Autodesk Inventor part; units mm, degrees
ref_plane "YZ Plane" through (0, 0, 0) normal (1, 0, 0) x (0, 1, 0)
ref_plane "XZ Plane" through (0, 0, 0) normal (0, 1, 0) x (-1, 0, 0)
ref_plane "XY Plane" through (0, 0, 0) normal (0, 0, 1) x (1, 0, 0)
sketch "Szkic1" plane through (0, 0, 0) normal (0, 0, 1) x (1, 0, 0)
  circle A0 centre (0, 0) radius 15
  circle A1 centre (0, 0) radius 5
  dimension "d0" = 30
  dimension "d1" = 10
extrude "Wyciągnięcie proste1" add sketch "Szkic1" along normal blind 14
sketch "Szkic2" plane through (0, 0, 14) normal (0, 0, 1) x (1, 0, 0)
  circle A0 centre (0, 0) radius 6.5
  circle A1 centre (0, 0) radius 13.5
  dimension "d4" = 13
  dimension "d5" = 27
extrude "Wyciągnięcie proste2" cut sketch "Szkic2" against normal blind 1
sketch "Szkic3" plane through (0, 0, 0) normal (0, 0, -1) x (-1, 0, 0)
  circle A0 centre (0, 0) radius 6.5
  circle A1 centre (0, 0) radius 13.5
  dimension "d8" = 13
  dimension "d9" = 27
extrude "Wyciągnięcie proste3" cut sketch "Szkic3" against normal blind 1
properties part number "Łożysko kulowe jednorzędowe 3200 2RS"
CAD build for the part. Positions are in the model's coordinates, mm. A direction names the side the tool comes from. Round coordinates to 2 decimals unless told otherwise and drop trailing zeros. Order: outer loops, then holes, each group sorted by start corner. A loop starts at its lowest first (then second) coordinate and runs counter-clockwise, first axis right, second up. Notation, with made-up numbers: (79.5, 44) -> (120.5, 44) arc R35 ccw to (120.5, 78) -> close; hole circle Ø8 at (68.5, 19.25). An arc over 180 degrees is marked (long way). Write item = value, one per line.
(1) Drill centre lines: L1, parallel to Y at x = 0, z = 13.65; L2, parallel to Y at x = 0, z = 7.25; L3, parallel to Z at x = -6.75, y = 6. Where is each one in solid material? Low to high.
Answers follow:
L1 = -15 to -13.5, -6.5 to -5, 5 to 6.5, 13.5 to 15
L2 = -15 to -5, 5 to 15
L3 = 1 to 13
(2) Cut at C-C (z = 5.75). Write the cut outline in (x, y), plus the area to 3 significant figures.
Answers follow:
outline = circle Ø30 at (0, 0); hole circle Ø10 at (0, 0)
area = 628 mm²
(3) Cut at D-D (x = -9.75). Write the cut outline in (y, z), plus the area to 3 significant figures.
Answers follow:
outline = (-11.4, 0) -> (-9.34, 0) -> (-9.34, 1) -> (9.34, 1) -> (9.34, 0) -> (11.4, 0) -> (11.4, 14) -> (9.34, 14) -> (9.34, 13) -> (-9.34, 13) -> (-9.34, 14) -> (-11.4, 14) -> close
area = 282 mm²
(4) 3-axis set-ups, long thin cutter, end or side, ignore diameter. For faces 4 (the cylindrical face through (-5.158, -3.955, 13.507)), 5 (the flat face through (2, -5, 0)), 6 (the cylindrical face through (2.93, -13.18, 0.49)): which of +Z, -Z, +X, -X, +Y, -Y reach the whole face in a straight line?
Answers follow:
face_4 = +Z
face_5 = -Z, +X, -X, +Y, -Y
face_6 = -Z
(5) Flat gauge pins, fed straight in: P1, Ø2, axis at x = -7.5, y = 3.5, coming from the +Z side; P2, Ø2, axis at y = 8, z = 4.5, coming from the -X side; P3, Ø1, axis at x = 9.5, z = 3.5, coming from the +Y side. Where does each tip first touch, or does it go through?
Answers follow:
P1 = 13
P2 = -13.27
P3 = 12
(6) Pull direction Y, two halves, no side cores. Call faces 1 (the flat face through (-6, 3, 1)), 2 (the cylindrical face through (-14.985, -0.66, 6.902)), 3 (the flat face through (2, -5, 14)): +Y half, -Y half, draft (parallel to the pull), parting line (faces both ways), or undercut.
Answers follow:
face_1 = undercut
face_2 = parting line
face_3 = draft
(7) Cut at A-A (y = 0). Write the cut outline in (x, z), plus the area to 3 significant figures.
Answers follow:
outline = (-15, 0) -> (-13.5, 0) -> (-13.5, 1) -> (-6.5, 1) -> (-6.5, 0) -> (-5, 0) -> (-5, 14) -> (-6.5, 14) -> (-6.5, 13) -> (-13.5, 13) -> (-13.5, 14) -> (-15, 14) -> close; (5, 0) -> (6.5, 0) -> (6.5, 1) -> (13.5, 1) -> (13.5, 0) -> (15, 0) -> (15, 14) -> (13.5, 14) -> (13.5, 13) -> (6.5, 13) -> (6.5, 14) -> (5, 14) -> close
area = 252 mm²
